Read the model definition and answer for the solid it produces. Units are mm, in the model's axes. Give positions to 0.01 mm unless a question says otherwise; leave off trailing zeros. Loops run counter-clockwise (first coordinate to the right, second up) from the corner with the lowest first, then second, coordinate; pieces in that order, holes last. Notation, with made-up numbers: (14, -17.5) - (32, -17.5) arc R33 cw to (32, 13.5) - close; hole circle Ø9 at (69.5, 15). An arc over 180 degrees is marked (long way). Write item = value, one per line.
```python
from build123d import *

# Parameters (mm, degrees)
F0_W     = 76.2
F0_H     = 101.6
F1_DEPTH = 12.7
F2_R     = 25.4


with BuildPart() as f1:
    # F0 (on Top) → F1 (new body)
    with BuildSketch(Plane.XY):
        with Locations((38.1, -50.8)):
            Rectangle(F0_W, F0_H)
    extrude(amount=-F1_DEPTH)

    # F2
    f2_edges = [f1.edges().sort_by_distance(p)[0] for p in [
        (0, 0, -6.35),
        (0, -101.6, -6.35),
    ]]
    fillet(f2_edges, radius=F2_R)


solid = f1.part
```
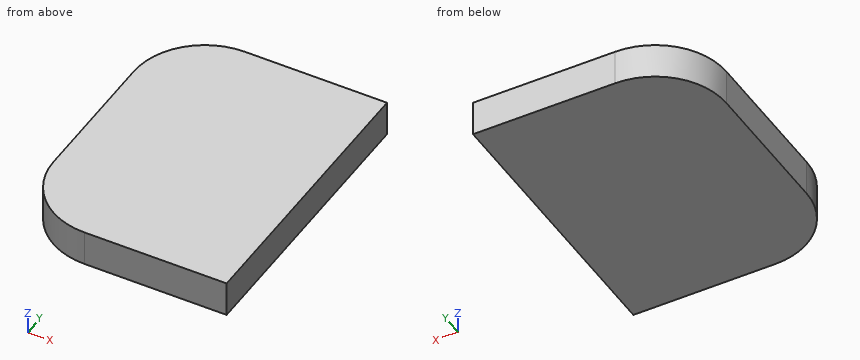
1) A cutting plane is placed at B-B on x = 14. Determine the outline of the cut face in (y, z).
Output:
outline = (-98.9, -12.7) - (-2.7, -12.7) - (-2.7, 0) - (-98.9, 0) - close
2) A cutting plane is placed at A-A on z = -5.5. Determine the outline of the cut face in (x, y).
Output:
outline = (0, -76.2) arc R25.4 ccw to (25.4, -101.6) - (76.2, -101.6) - (76.2, 0) - (25.4, 0) arc R25.4 ccw to (0, -25.4) - close
3) This flat-tipped pin is pushed along its axis until it touches: P1, Ø1, axis at x = 31, y = -67, coming from the +Z side. Where does it stop, or does it pass through?
Output:
P1 = 0
4) Find the intervals of material crossed by probe 1 along Y at (x, z) = (25, -11); probe 2 along X at (y, z) = (-89, -3.5); probe 3 along X at (y, z) = (-92, -6), in increasing order.
Output:
probe_1 = -101.6 to 0
probe_2 = 3.46 to 76.2
probe_3 = 5.51 to 76.2
